Read the model definition and answer for the solid it produces. Units are mm, in the model's axes. A direction names the side the tool comes from. Round coordinates to 2 decimals unless told otherwise and drop trailing zeros. Write each loop counter-clockwise with the first axis right and the second up, starting at its lowest first coordinate (ties: lowest second). Pieces come first, ordered by that corner, then holes. Notation, with made-up numbers: M -18,4 L 1,4 A34 ccw 1,41 Z; hole C 63,-25 d7. An arc over 180 degrees is marked long. Use one line per item in the form item = value. Start each with the question number.
```python
from build123d import *

# Parameters (mm, degrees)
F1_DEPTH = 850
F2_W     = 550
F2_H     = 150
F4_DEPTH = 600
F2_W_2   = 500
F2_H_2   = 750
F5_DEPTH = 10
F3_W     = 500
F3_H     = 750
F8_DEPTH = 10


with BuildPart() as f1:
    # F0 (on Top) → F1 (new body)
    with BuildSketch(Plane.XY):
        with BuildLine():
            Line((-2400, 0), (0, 0))
            Line((0, 0), (0, 1350))
            Line((0, 1350), (-550, 1350))
            ThreePointArc((-550, 1350), (-620.710678, 1320.710678), (-650, 1250))
            Line((-650, 1250), (-650, 650))
            Line((-650, 650), (-2400, 650))
            ThreePointArc((-2400, 650), (-2470.710678, 620.710678), (-2500, 550))
            Line((-2500, 550), (-2500, 100))
            ThreePointArc((-2500, 100), (-2470.710678, 29.289322), (-2400, 0))
        make_face()
    extrude(amount=F1_DEPTH)

    # F2 (on face) → F4 (cut)
    with BuildSketch(Plane(origin=(0, 650, 0), x_dir=(-1, 0, 0), z_dir=(0, 1, 0))):
        with Locations((975, 725)):
            Rectangle(F2_W, F2_H)
        with Locations((975, 525)):
            Rectangle(F2_W, F2_H)
        with Locations((975, 325)):
            Rectangle(F2_W, F2_H)
        with Locations((975, 125)):
            Rectangle(F2_W, F2_H)
    extrude(amount=-F4_DEPTH, mode=Mode.SUBTRACT)

    # F2 (on face) → F5 (join)
    with BuildSketch(Plane(origin=(0, 650, 0), x_dir=(-1, 0, 0), z_dir=(0, 1, 0))):
        with Locations((1550, 425)):
            Rectangle(F2_W_2, F2_H_2)
        with Locations((2100, 425)):
            Rectangle(F2_W_2, F2_H_2)
    extrude(amount=F5_DEPTH)

    # F3 (on face) → F8 (join)
    with BuildSketch(Plane(origin=(-650, 0, 0), x_dir=(0, -1, 0), z_dir=(-1, 0, 0))):
        with Locations((-950, 425)):
            Rectangle(F3_W, F3_H)
    extrude(amount=F8_DEPTH)


solid = f1.part
```
Q1. Find section A-A on y = 247. Write down the section's boundary in (x, z).
Q2. Each of these flat-tipped pins is pushed along its axis until it touches: pin 1 Ø5 at (x, y) = (-1983, 653.5) entering from -Z; pin 2 Ø5 at (y, z) = (930.5, 278.5) entering from -X; pin 3 Ø3 at (y, z) = (656.5, 557) entering from -X. Where does it stop, or does it pass through?
Q3. Straight lines are drawn through the part: line 1 (Z direction, x = -855, y = 142); line 2 (X direction, y = 367.5, z = 738.5); line 3 (Y direction, x = -929.5, z = 762). For each, find the intervals that lie inside material, in ascending order. Write a range as [from, to].
Q4. Find section D-D on y = 739.5. Write down the section's boundary in (x, z), and give its area (3 significant figures).
Q5. For a pull along Z with two mould halves and no side action, classify faces 1 (the face through (-2469.929, 621.484, 419.05)), 2 (the face through (-990, 384, 0)), 3 (the face through (-971, 354, 800)) as +Z half, -Z half, draft (parallel to the pull), parting line (faces both ways), or undercut.
Q6. Find section C-C on z = 276. Write down the section's boundary in (x, y), and give its area (3 significant figures).
Q7. A tool of negligible diameter and unlimited length cuts with its end or side. For faces 4 (the face through (-271, 1350, 419)), 5 (the face through (-1250, 354, 324)), 6 (the face through (-660, 954, 430)), from which of +Z, -Z, +X, -X, +Y, -Y can it reach the whole face along a straight path? Write none if from no direction.
Q8. Find section B-B on x = -2079. Write down the section's boundary in (y, z), and give its area (3 significant figures).
Response:
q1.outline = M -2500,0 L 0,0 L 0,850 L -2500,850 Z; hole M -1250,50 L -700,50 L -700,200 L -1250,200 Z; hole M -1250,250 L -700,250 L -700,400 L -1250,400 Z; hole M -1250,450 L -700,450 L -700,600 L -1250,600 Z; hole M -1250,650 L -700,650 L -700,800 L -1250,800 Z
q2.pin_1 = 50
q2.pin_2 = -660
q2.pin_3 = -2350
q3.line_1 = [0, 50], [200, 250], [400, 450], [600, 650], [800, 850]
q3.line_2 = [-2500, -1250], [-700, 0]
q3.line_3 = [0, 50]
q4.outline = M -660,50 L -650,50 L -650,0 L 0,0 L 0,850 L -650,850 L -650,800 L -660,800 Z
q4.area = 560,000 mm²
q5.face_1 = draft
q5.face_2 = -Z half
q5.face_3 = undercut
q6.outline = M -2500,100 A100 ccw -2400,0 L 0,0 L 0,1350 L -550,1350 A100 ccw -650,1250 L -650,1200 L -660,1200 L -660,700 L -650,700 L -650,650 L -700,650 L -700,50 L -1250,50 L -1250,650 L -1300,650 L -1300,660 L -1800,660 L -1800,650 L -1850,650 L -1850,660 L -2350,660 L -2350,650 L -2400,650 A100 ccw -2500,550 Z
q6.area = 1,760,000 mm²
q7.face_4 = +Z, -Z, +X, -X, +Y
q7.face_5 = +Y
q7.face_6 = +Z, -Z, -X, +Y
q8.outline = M 0,0 L 650,0 L 650,50 L 660,50 L 660,800 L 650,800 L 650,850 L 0,850 Z
q8.area = 560,000 mm²
